The model under review builds one solid part; all positions refer to its coordinate system, in mm. A direction names the side the tool comes from. Give positions to 0.01 mm unless a question says otherwise; leave off trailing zeros. Order: outer loops, then holes, each group sorted by start corner. A loop starts at its lowest first (then second) coordinate and runs counter-clockwise, first axis right, second up. Notation, with made-up numbers: (9, 2.25) - (33, 2.25) arc R5 cw to (33, 10.25) - close; hole circle Ø10 at (42, -38). An arc over 180 degrees is marked (long way). Put each result on its own line as item: value.
```python
from build123d import *

# Parameters (mm, degrees)
F1_DEPTH = 50.8
F2_W     = 25.4
F2_H     = 25.4
F2_H_2   = 12.7
F2_R     = 3.175
F3_DEPTH = 11.5072
F4_R     = 3.2131
F5_DEPTH = 88.901


with BuildPart() as f1:
    # F0 (on Top) → F1 (new body, symmetric)
    with BuildSketch(Plane.XY):
        with BuildLine():
            Line((-36.7919, -5.7531), (0, -5.7531))
            ThreePointArc((0, -5.7531), (2.703042, 5.078555), (-4.772227, -3.2131))
            Line((-4.772227, -3.2131), (-36.7919, -3.2131))
            Line((-36.7919, -3.2131), (-36.7919, -5.7531))
        make_face()
    extrude(amount=F1_DEPTH, both=True)

    # F2 (on face) → F3 (cut, through all)
    with BuildSketch(Plane.XZ.offset(5.7531)):
        with Locations((5.4991, 0)):
            Rectangle(F2_W, F2_H)
        with Locations((5.4991, 44.45)):
            Rectangle(F2_W, F2_H_2)
        with Locations((5.4991, -44.45)):
            Rectangle(F2_W, F2_H_2)
        with Locations((-24.0919, 25.4)):
            Circle(F2_R)
        with Locations((-24.0919, -25.4)):
            Circle(F2_R)
    extrude(amount=-F3_DEPTH, mode=Mode.SUBTRACT)

    # F4 (on face) → F5 (cut, through all)
    with BuildSketch(Plane.XY.offset(38.1)):
        Circle(F4_R)
    extrude(amount=-F5_DEPTH, mode=Mode.SUBTRACT)


solid = f1.part
```
(1) Take a section at C-C, the plane x = -22.5. Write out the cut boundary in (y, z).
The answers:
outline: (-5.75, -50.8) - (-3.21, -50.8) - (-3.21, -28.15) - (-5.75, -28.15) - close; (-5.75, -22.65) - (-3.21, -22.65) - (-3.21, 22.65) - (-5.75, 22.65) - close; (-5.75, 28.15) - (-3.21, 28.15) - (-3.21, 50.8) - (-5.75, 50.8) - close
(2) Clearance check with flat-ended pins moving along their axes: pin 1 Ø1.5 at (y, z) = (0.5, -34) entering from -X; pin 2 Ø1.3 at (y, z) = (-5, 42.5) entering from +X; pin 3 Ø7.5 at (x, z) = (-24.09, -25.4) entering from +Y. State where each tip first meets the part, or that it passes through.
The answers:
pin 1: x = -5.75
pin 2: x = -7.2
pin 3: y = -3.21
(3) Take a section at B-B, the plane y = 0. Write out the cut boundary in (x, z).
The answers:
outline: (-5.75, -38.1) - (-3.21, -38.1) - (-3.21, -12.7) - (-5.75, -12.7) - close; (-5.75, 12.7) - (-3.21, 12.7) - (-3.21, 38.1) - (-5.75, 38.1) - close; (3.21, -38.1) - (5.75, -38.1) - (5.75, -12.7) - (3.21, -12.7) - close; (3.21, 12.7) - (5.75, 12.7) - (5.75, 38.1) - (3.21, 38.1) - close
(4) Take a section at D-D, the plane y = 4.75. Write out the cut boundary in (x, z), then the cut area to 3 significant figures.
The answers:
outline: (-3.25, -38.1) - (3.25, -38.1) - (3.25, -12.7) - (-3.25, -12.7) - close; (-3.25, 12.7) - (3.25, 12.7) - (3.25, 38.1) - (-3.25, 38.1) - close
area: 330 mm^2
(5) The part is to be moulded in two halves that separate along X. For faces 6 (the cylindrical face through (-3.21, 0.14, -25.22)), 7 (the flat face through (-7.201, -5, 44)), 8 (the cylindrical face through (-24.505, -4.501, -22.252)), 9 (the flat face through (-2, -3, -12.7)), say which applies: pulls with the +X half, pulls with the -X half, needs draft (parallel to the pull), parting line crosses it, or undercut.
The answers:
face 6: undercut
face 7: pulls with the +X half
face 8: undercut
face 9: needs draft
(6) Wall thickness on L1, parallel to Z at x = -4, y = -2.25; L2, parallel to Z at x = -26.5, y = -4; L3, parallel to Y at x = 0, z = -17.75: over which ranges is each line inside the solid? List them lowest first.
The answers:
L1: -38.1 to -12.7, 12.7 to 38.1
L2: -50.8 to -27.47, -23.33 to 23.33, 27.47 to 50.8
L3: -5.75 to -3.21, 3.21 to 5.75
(7) For faces 1 (the flat face through (-2, -3, 38.1)), 2 (the flat face through (-2, -3, 12.7)), 3 (the flat face through (-19, -5.753, 1)), 4 (the cylindrical face through (-3.21, 0.14, 25.58)), 5 (the flat face through (-2, -3, -38.1)), list the 3-axis set-ups (+Z, -Z, +X, -X, +Y, -Y) from which the entire face can be reached by the end or side of a thin tool; tool diameter is ignored.
The answers:
face 1: +Z, +X, +Y, -Y
face 2: +X, +Y, -Y
face 3: +Z, -Z, +X, -X, -Y
face 4: +Z, -Z
face 5: -Z, +X, +Y, -Y
(8) Take a section at A-A, the plane z = 25.4. Write out the cut boundary in (x, y), then the cut area to 3 significant figures.
The answers:
outline: (-36.79, -5.75) - (-27.27, -5.75) - (-27.27, -3.21) - (-36.79, -3.21) - close; (-20.92, -5.75) - (0, -5.75) arc R5.75 ccw (long way) to (-4.77, -3.21) - (-20.92, -3.21) - close; hole circle Ø6.43 at (0, 0)
area: 140 mm^2
